Check sheet for the modelled part. Datum: model origin and axes. Units: mm. Face numbers are marked on the shaded views. A direction names the side the tool comes from. Round coordinates to 2 decimals unless told otherwise and drop trailing zeros. Write each loop counter-clockwise with the first axis right and the second up, starting at its lowest first coordinate (ties: lowest second). Pieces come first, ordered by that corner, then holes. Notation, with made-up numbers: M 71,-27.75 L 129,-27.75 A17 ccw 129,1.25 Z; hole C -26,48.25 d8. An arc over 180 degrees is marked long. Put each result on its own line as item: value.
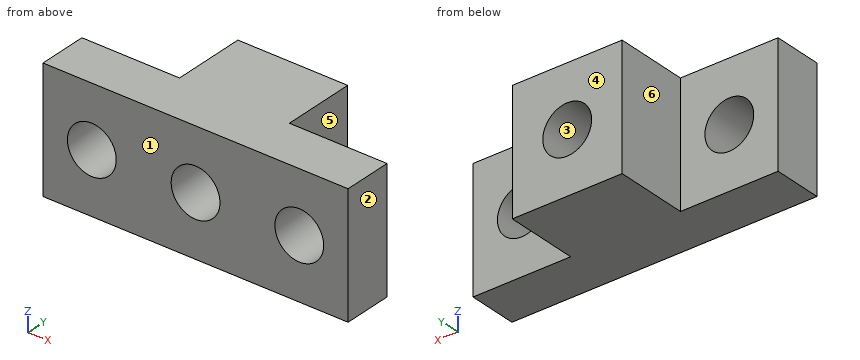
```python
from build123d import *

# Parameters (mm, degrees)
SKETCH1_W           = 25
SKETCH1_H           = 10
BOSS_EXTRUDE1_DEPTH = 10
SKETCH2_W           = 8
SKETCH2_H           = 6
CUT_EXTRUDE1_DEPTH  = 10
SKETCH3_R           = 2
CUT_EXTRUDE2_DEPTH  = 17.770509831
SKETCH4_R           = 2
CUT_EXTRUDE3_DEPTH  = 10


with BuildPart() as part:
    # Sketch1 → Boss-Extrude1 (new body)
    with BuildSketch(Plane(origin=(0, 0, 0), x_dir=(1, 0, 0), z_dir=(0, 1, 0))):
        Rectangle(SKETCH1_W, SKETCH1_H)
    extrude(amount=BOSS_EXTRUDE1_DEPTH)

    # Sketch2 → Cut-Extrude1 (cut)
    with BuildSketch(Plane.XY.offset(5)):
        with Locations((-8.5, 7)):
            Rectangle(SKETCH2_W, SKETCH2_H)
        with Locations((8.5, 7)):
            Rectangle(SKETCH2_W, SKETCH2_H)
    extrude(amount=-CUT_EXTRUDE1_DEPTH, mode=Mode.SUBTRACT)

    # Sketch3 → Cut-Extrude2 (cut, through all)
    with BuildSketch(Plane(origin=(0, 10, 0), x_dir=(1, 0, 0), z_dir=(0, 1, 0))):
        with Locations(Location((0, 0, 0), (0, 0, 270))):
            Circle(SKETCH3_R)
    extrude(amount=-CUT_EXTRUDE2_DEPTH, mode=Mode.SUBTRACT)

    # Sketch4 → Cut-Extrude3 (cut)
    with BuildSketch(Plane(origin=(0, 4, 0), x_dir=(1, 0, 0), z_dir=(0, 1, 0))):
        with Locations(Location((-8.5, 0, 0), (0, 0, 270))):
            Circle(SKETCH4_R)
        with Locations(Location((8.5, 0, 0), (0, 0, 270))):
            Circle(SKETCH4_R)
    extrude(amount=-CUT_EXTRUDE3_DEPTH, mode=Mode.SUBTRACT)


solid = part.part
```
1. Cross-section at C-C (z = 3.5). Enter the section's corners in (x, y).
Computed values:
outline: M -12.5,0 L 12.5,0 L 12.5,4 L 4.5,4 L 4.5,10 L -4.5,10 L -4.5,4 L -12.5,4 Z
2. Release check for a two-part mould opening along X. For the marked faces 1, 2 and 3 record: +X half, -X half, draft (parallel to the pull), parting line (faces both ways), or undercut.
Computed values:
face 1: draft
face 2: +X half
face 3: undercut
3. Scan lines: probe 1 along X at (y, z) = (2.4, 0); probe 2 along X at (y, z) = (1.75, 1.25); probe 3 along Y at (x, z) = (6.5, 3). Record each from-to range of solid material in increasing order.
Computed values:
probe 1: x = -12.5 to -10.5, -6.5 to -2, 2 to 6.5, 10.5 to 12.5
probe 2: x = -12.5 to -10.06, -6.94 to -1.56, 1.56 to 6.94, 10.06 to 12.5
probe 3: y = 0 to 4
4. Cross-section at A-A (x = 8.5). Enter the section's corners in (y, z).
Computed values:
outline: M 0,-5 L 4,-5 L 4,-2 L 0,-2 Z; M 0,2 L 4,2 L 4,5 L 0,5 Z
5. Depth check by flat-ended pin: pin 1 Ø5 at (y, z) = (8, -2.5) entering from -X; pin 2 Ø5 at (y, z) = (7.5, -2.5) entering from +X; pin 3 Ø4 at (x, z) = (10.5, 0.5) entering from +Y. Enter the tip coordinate at first touch or a pass-through.
Computed values:
pin 1: stops at x = -4.5
pin 2: stops at x = 4.5
pin 3: stops at y = 4
6. Cross-section at D-D (y = 4.5). Enter the section's corners in (x, z).
Computed values:
outline: M -4.5,-5 L 4.5,-5 L 4.5,5 L -4.5,5 Z; hole C 0,0 d4
7. Access from +Z, -Z, +X, -X, +Y, -Y to the whole of each face (thin tool, end or side, straight path). Record for the marked faces 4, 5 and 6.
Computed values:
face 4: +Z, -Z, +X, -X, +Y
face 5: +Z, -Z, +X, +Y
face 6: +Z, -Z, -X, +Y
8. Cross-section at B-B (y = 2). Enter the section's corners in (x, z).
Computed values:
outline: M -12.5,-5 L 12.5,-5 L 12.5,5 L -12.5,5 Z; hole C -8.5,0 d4; hole C 0,0 d4; hole C 8.5,0 d4
